Work out the finished part from the listing and answer in its coordinate system (mm). A direction names the side the tool comes from. Round coordinates to 2 decimals unless told otherwise and drop trailing zeros. Write each loop counter-clockwise with the first axis right and the second up, starting at its lowest first coordinate (ties: lowest second). Pieces come first, ordered by that corner, then holes. Notation, with made-up numbers: (-9, -16.75) - (24, -16.75) arc R12 ccw to (24, 1.25) - close; hole circle Ø10 at (25, -39.5). An arc over 180 degrees is marked (long way). Write item = value, one per line. Start each with the question number.
from build123d import *

# Parameters (mm, degrees)
SKETCH2_R          = 3
CUT_EXTRUDE1_DEPTH = 10
CIRPATTERN1_COUNT  = 6


with BuildPart() as part:
    # Sketch1 → Revolve1 (revolve)
    with BuildSketch(Plane.XY):
        Polygon((0, 35), (5, 35), (5, 21), (8, 21), (8, 16), (5, 16), (5, 0), (0, 0), align=None)
    revolve(axis=Axis((5, 0, 0), (-1, 0, 0)))

    # Sketch2 → Cut-Extrude1 (cut)
    with BuildSketch(Plane(origin=(5, 0, 0), x_dir=(0, 0, -1), z_dir=(1, 0, 0))):
        with Locations((27.5, 0)):
            Circle(SKETCH2_R)
    cut_extrude1 = extrude(amount=-CUT_EXTRUDE1_DEPTH, mode=Mode.SUBTRACT)

    # CirPattern1: Cut-Extrude1 ×6 about axis
    cirpattern1_axis = Axis((0, 0, 0), (1, 0, 0))
    for i in range(1, CIRPATTERN1_COUNT):
        add(cut_extrude1.rotate(cirpattern1_axis, i * 360 / CIRPATTERN1_COUNT), mode=Mode.SUBTRACT)


solid = part.part
1. Find section D-D on x = 1. Give the vertices of the cut face in (y, z), plus the area to 3 significant figures.
2. For a pull along Z with two mould halves and no side action, classify faces 1 (the face through (5, 0, 0)), 2 (the face through (6.52, 20.03, -6.31)), 3 (the face through (8, -4.8, 15.5)) as released by +Z, released by -Z, zero draft, split by the parting line, or undercut.
3. Find section A-A on y = 0. Give the vertices of the cut face in (x, z).
4. Each of these flat-tipped pins is pushed along its axis until it touches: pin 1 (4 mm diameter, centred on x = 5, y = 26, fed in from +Z); pin 2 (9.5 mm diameter, centred on y = 0, z = -27.5, fed in from -X); pin 3 (5.5 mm diameter, centred on y = 0, z = 27.5, fed in from -X); pin 4 (2 mm diameter, centred on y = -7.5, z = -23.5, fed in from +X). Where does it stop, or does it pass through?
5. Consider line 1 (Y direction, x = 3.25, z = -11); line 2 (Z direction, x = 2.25, y = 1.5); line 3 (Y direction, x = 4.25, z = 13). Determine where each line is inside the solid, lowest interval first.
6. Which of the six approach directions +Z, -Z, +X, -X, +Y, -Y give full straight-line access (tool end or side, diameter ignored) to faces 4 (the face through (6.48, -3.47, 15.62)), 5 (the face through (2.5, 0.1, -24.5))?
7. Find section C-C on z = 13.75. Give the vertices of the cut face in (x, y), plus the area to 3 significant figures.
8. Find section B-B on z = 26.5. Give the vertices of the cut face in (x, y).
Answer key:
q1.outline = circle Ø70 at (0, 0); hole circle Ø6 at (-23.82, -13.75); hole circle Ø6 at (-23.82, 13.75); hole circle Ø6 at (0, -27.5); hole circle Ø6 at (0, 27.5); hole circle Ø6 at (23.82, -13.75); hole circle Ø6 at (23.82, 13.75)
q1.area = 3,680 mm²
q2.face_1 = undercut
q2.face_2 = split by the parting line
q2.face_3 = zero draft
q3.outline = (0, -35) - (5, -35) - (5, -30.5) - (0, -30.5) - close; (0, -24.5) - (5, -24.5) - (5, -21) - (8, -21) - (8, -16) - (5, -16) - (5, 16) - (8, 16) - (8, 21) - (5, 21) - (5, 24.5) - (0, 24.5) - close; (0, 30.5) - (5, 30.5) - (5, 35) - (0, 35) - close
q4.pin_1 = 25.48
q4.pin_2 = 0
q4.pin_3 = through
q4.pin_4 = 5
q5.line_1 = -33.23 to -25.01, -22.62 to 22.62, 25.01 to 33.23
q5.line_2 = -34.97 to -30.1, -24.9 to 24.9, 30.1 to 34.97
q5.line_3 = -32.5 to -26.72, -20.91 to 20.91, 26.72 to 32.5
q6.face_4 = +X
q6.face_5 = +X, -X
q7.outline = (0, -32.19) - (5, -32.19) - (5, -26.82) - (0, -26.82) - close; (0, -20.82) - (5, -20.82) - (5, -15.87) - (8, -15.87) - (8, -8.18) - (5, -8.18) - (5, 8.18) - (8, 8.18) - (8, 15.87) - (5, 15.87) - (5, 20.82) - (0, 20.82) - close; (0, 26.82) - (5, 26.82) - (5, 32.19) - (0, 32.19) - close
q7.area = 308 mm²
q8.outline = (0, -22.86) - (5, -22.86) - (5, -2.83) - (0, -2.83) - close; (0, 2.83) - (5, 2.83) - (5, 22.86) - (0, 22.86) - close
